Could you check a few things on this model? Use its own coordinates, in mm. A direction names the side the tool comes from. Round coordinates to 2 decimals unless told otherwise and drop trailing zeros. Write each loop counter-clockwise with the first axis right and the second up, starting at its lowest first coordinate (ties: lowest second). Pieces come first, ordered by that corner, then holes. Notation, with made-up numbers: (-37, -17.75) -> (-31, -17.75) arc R33 cw to (-31, 14.25) -> close; hole circle Ø5 at (-13, -39.5). An arc over 180 degrees is marked (long way). Answer in a Markdown table with one row per item. Add a question column.
Autodesk Inventor part; units mm, degrees
ref_plane "YZ Plane" through (0, 0, 0) normal (1, 0, 0) x (0, 1, 0)
ref_plane "XZ Plane" through (0, 0, 0) normal (0, 1, 0) x (-1, 0, 0)
ref_plane "XY Plane" through (0, 0, 0) normal (0, 0, 1) x (1, 0, 0)
sketch "Skizze1" plane through (0, 0, 0) normal (0, 0, 1) x (1, 0, 0)
  line L0 (0, 0) -> (85, 0)
  line L1 (85, 0) -> (85, 95)
  line L2 (85, 95) -> (0, 95)
  line L3 (0, 95) -> (0, 0)
  dimension "d0" = 85
  dimension "d1" = 95
extrude "Extrusion1" add sketch "Skizze1" along normal blind 80
sketch "Skizze2" plane through (85, 0, 0) normal (1, 0, 0) x (0, 0, -1)
  line L0 (0, 0) -> (-80, 0)
  line L1 (0, 0) -> (-15, 0)
  line L2 (-15, 0) -> (-55, 69.282)
  line L3 (-55, 69.282) -> (-55, 95)
  line L4 (0, 95) -> (-80, 95)
  line L5 (-55, 95) -> (0, 95)
  line L6 (0, 0) -> (0, 95)
  line L7 (0, 95) -> (0, 0)
  line L8 (0, 95) -> (0, 0)
  dimension "d4" = 15
  dimension "d5" = 80
  dimension "d6" = 120
extrude "Extrusion2" cut sketch "Skizze2" against normal through all keep common part
sketch "Skizze3" plane through (0, 0, 15) normal (0, -0.5, 0.866) x (1, 0, 0)
  line L0 (5.5, 72.5) -> (79.5, 72.5)
  line L1 (79.5, 72.5) -> (79.5, 8)
  line L2 (79.5, 8) -> (5.5, 8)
  line L3 (5.5, 8) -> (5.5, 72.5)
  line L4 (85, -7.5) -> (85, 74.7724)
  line L5 (85, 80) -> (0, 80)
  line L6 (0, 0) -> (85, 0)
  point P0 (0, -7.5)
  point P1 (79.5, 40.25)
  point P2 (42.5, 72.5)
  point P3 (42.5, 80)
  dimension "d9" = 74
  dimension "d10" = 64.5
  dimension "d13" = 8
extrude "Extrusion3" cut sketch "Skizze3" against normal blind 16.36
sketch "Skizze4" plane through (79.5, 6.9282, 19) normal (-1, 0, 0) x (0, -0.5, 0.866)
  line L0 (-12.26, 3.15) -> (-1.46, 3.15)
  line L1 (-1.46, 3.15) -> (-1.46, 15.35)
  line L2 (-1.46, 15.35) -> (-12.26, 15.35)
  line L3 (-12.26, 15.35) -> (-12.26, 3.15)
  line L4 (-16.36, 64.5) -> (-16.36, 0)
  line L5 (0, 0) -> (-16.36, 0)
  line L6 (0, 64.5) -> (0, 0)
  point P0 (-12.9904, -15.5)
  dimension "d15" = 4.1
  dimension "d16" = 3.15
  dimension "d17" = 12.2
  dimension "d18" = 10.8
  dimension "d19" = 1.46
extrude "Extrusion4" cut sketch "Skizze4" against normal through all
fillet "Rundung2" radius 1.5 4 edges at (82.25, 26.3517, 16.0575) (82.25, 15.7862, 9.9575) (82.25, 10.3862, 19.3106) (82.25, 20.9517, 25.4106)
sketch "Skizze6" plane through (0, 0, 15) normal (0, -0.5, 0.866) x (1, 0, 0)
  circle A0 centre (4, 4) radius 2.25
  circle A1 centre (4, 76) radius 2.25
  circle A2 centre (81, 76) radius 2.25
  circle A3 centre (81, 4) radius 2.25
  point P0 (0, -7.5)
hole "Bohrung2" at (81, 3.4641, 17) at (81, 65.8179, 53) at (4, 65.8179, 53) at (4, 3.4641, 17) direction (0, 0.5, -0.866) diameter 3.242 depth 11.8 tip angle 118
sketch "Skizze7" plane through (0, 95, 0) normal (0, 1, 0) x (1, 0, 0)
  line L0 (85, -55) -> (0, -55)
  line L1 (85, 0) -> (85, -55)
  line L2 (85, 0) -> (0, 0)
  line L3 (0, 0) -> (0, -55)
  line L4 (85, 0) -> (85, -55)
  line L5 (85, -55) -> (42.5, -55)
  line L6 (42.5, -55) -> (42.5, -41)
  line L7 (42.5, -41) -> (85, -41)
  line L8 (85, -41) -> (85, -55)
  point P0 (0, 0)
  dimension "d37" = 42.5
  dimension "d38" = 14
hole "Bohrung3" at (42.5, 95, 41) direction (0, -1, 0) diameter 10 end through all
sketch "Skizze8" plane through (0, 8.18, 0.8318) normal (0, -0.5, 0.866) x (1, 0, 0)
  circle A0 centre (11.65, 13) radius 1.6
  circle A1 centre (74.16, 11.255) radius 1.165
  circle A2 centre (73.65, 67) radius 1.6
  circle A3 centre (11.65, 67) radius 1.6
  circle A4 centre (57.65, 13) radius 1.6
  point P0 (0, -7.5)
hole "Bohrung4" at (57.65, 19.4383, 7.3318) at (11.65, 19.4383, 7.3318) at (11.65, 66.2037, 34.3318) at (73.65, 66.2037, 34.3318) direction (0, 0.5, -0.866) diameter 2.459 depth 7 tip angle 118
sketch "Skizze9" plane through (0, 95, 0) normal (0, 1, 0) x (1, 0, 0)
  line L0 (72.5, -48) -> (12.5, -48)
  line L1 (12.5, -48) -> (12.5, -7)
  line L2 (12.5, -7) -> (72.5, -7)
  line L3 (72.5, -7) -> (72.5, -48)
  line L4 (85, -55) -> (0, -55)
  line L5 (85, 0) -> (0, 0)
  point P0 (42.5, -48)
  point P1 (42.5, -55)
  dimension "d54" = 60
  dimension "d55" = 41
  dimension "d56" = 7
  dimension "d57" = 7
hole "Bohrung5" at (12.5, 95, 48) at (12.5, 95, 7) at (72.5, 95, 7) at (72.5, 95, 48) direction (0, -1, 0) diameter 4.917 depth 20 tip angle 118
fillet "Rundung3" radius 1.5 4 edges at (0, 95, 27.5) (0, 0, 7.5) (85, 0, 7.5) (85, 95, 27.5)
fillet "Rundung1" radius 3.1 4 edges at (5.5, 66.8773, 44.165) (79.5, 66.8773, 44.165) (79.5, 11.0187, 11.915) (5.5, 11.0187, 11.915)
properties part number "Gehause"
(1) Suppose I cut it at B-B, the plane x = 66. Please give me the cut outline in (y, z).
(2) Suppose I cut it at A-A, the plane y = 81.5. Please give me the cut outline in (x, z), then the cut area to 3 significant figures.
(3) For P1, Ø21.5, axis at y = 45, z = 31.5, coming from the -X side; P2, Ø4.5, axis at x = 12.5, z = 48, coming from the -Y side; P3, Ø4.5, axis at x = 72.5, z = 48, coming from the +Y side; P4, Ø1, axis at x = 32.5, z = 16.5, coming from the -Y side, each with a flat end and sliding along its axis, tell me the tip position at first contact or that it passes through.
(4) I need wall thicknesses on L1, parallel to X at y = 86.5, z = 48; L2, parallel to Z at x = 12.5, y = 91.25; L3, parallel to X at y = 40, z = 28. Which ranges of each line are inside material? Lowest first, please.
(5) If we mould it in two halves opening along X, with no side actions, what happens to faces 5 (the face through (82.212, 21.125, 13.04)), 6 (the face through (0, 58, 21)), 7 (the face through (78.616, 11.883, 12.282))? For each: pulls with the +X half, pulls with the -X half, needs draft (parallel to the pull), parting line crosses it, or undercut.
(6) Suppose I cut it at C-C, the plane z = 23. Please give me the cut outline in (x, y), then the cut area to 3 significant figures.
(7) Suppose I cut it at D-D, the plane x = 42.5. Please give me the cut outline in (y, z), then the cut area to 3 significant figures.
(8) On a 3-axis mill with a long thin cutter (end or side, diameter ignored), from which of +Z, -Z, +X, -X, +Y, -Y can I reach the whole of each face in a straight line? I mean faces 1 (the face through (42.975, 10.961, 12.014)), 2 (the face through (4.24, 9.64, 6.01)), 3 (the face through (10.062, 84.86, 6.68)), 4 (the face through (82.212, 15.613, 22.328)). Say none if no direction works.
Response:
| question | item | result |
|---|---|---|
| 1 | outline | (0, 0) -> (95, 0) -> (95, 55) -> (69.28, 55) -> (62.79, 51.25) -> (70.97, 37.08) -> (15.11, 4.83) -> (6.93, 19) -> (0, 15) -> close |
| 2 | outline | (0, 0) -> (85, 0) -> (85, 55) -> (0, 55) -> close; hole circle Ø4.92 at (12.5, 7); hole circle Ø4.92 at (12.5, 48); hole circle Ø10 at (42.5, 41); hole circle Ø4.92 at (72.5, 7); hole circle Ø4.92 at (72.5, 48) |
| 2 | area | 4,520 mm² |
| 3 | P1 | x = 0 |
| 3 | P2 | y = 63.36 |
| 3 | P3 | y = 74.87 |
| 3 | P4 | y = 1.73 |
| 4 | L1 | 0 to 10.04, 14.96 to 70.04, 74.96 to 85 |
| 4 | L2 | 0 to 4.54, 9.46 to 45.54, 50.46 to 55 |
| 4 | L3 | 0 to 5.5, 79.5 to 85 |
| 5 | face 5 | needs draft |
| 5 | face 6 | pulls with the -X half |
| 5 | face 7 | undercut |
| 6 | outline | (0, 13.86) -> (5.5, 13.86) -> (5.5, 46.58) -> (79.5, 46.58) -> (79.5, 22.34) -> (85, 22.34) -> (85, 93.5) arc R1.5 ccw to (83.5, 95) -> (1.5, 95) arc R1.5 ccw to (0, 93.5) -> close; (79.5, 13.86) -> (85, 13.86) -> (85, 16.78) -> (79.5, 16.78) -> close |
| 6 | area | 4,440 mm² |
| 7 | outline | (0, 0) -> (95, 0) -> (95, 36) -> (69.1, 36) -> (15.11, 4.83) -> (6.93, 19) -> (0, 15) -> close; (62.79, 51.25) -> (65.82, 46) -> (95, 46) -> (95, 55) -> (69.28, 55) -> close |
| 7 | area | 2,520 mm² |
| 8 | face 1 | +Z |
| 8 | face 2 | none |
| 8 | face 3 | +Y |
| 8 | face 4 | +X |
